Design review of the part built by this model. Coordinates are the model's own, in mm. A direction names the side the tool comes from. Give positions to 0.01 mm unless a question says otherwise; leave off trailing zeros. Write each loop counter-clockwise with the first axis right and the second up, starting at its lowest first coordinate (ties: lowest second). Pieces come first, ordered by that corner, then holes.
```python
from build123d import *

# Parameters (mm, degrees)
SKETCH1_W           = 1.5875
SKETCH1_H           = 40
SKETCH1_W_2         = 6.825
BOSS_EXTRUDE1_DEPTH = 1.5875
SKETCH1_3_W         = 1.5875
SKETCH1_3_H         = 40
BOSS_EXTRUDE2_DEPTH = 25
SKETCH2_W           = 10
SKETCH2_H           = 8
CUT_EXTRUDE1_DEPTH  = 11


with BuildPart() as part:
    # Sketch1 → Boss-Extrude1 (new body)
    with BuildSketch(Plane(origin=(0, 0, 0), x_dir=(1, 0, 0), z_dir=(0, 1, 0))):
        with Locations((-4.20625, 0)):
            Rectangle(SKETCH1_W, SKETCH1_H)
        Rectangle(SKETCH1_W_2, SKETCH1_H)
        with BuildLine():
            ThreePointArc((2.75, -10), (-1.944543648, -11.944543648), (0, -7.25))
            ThreePointArc((0, -7.25), (1.944543648, -8.055456352), (2.75, -10))
        make_face(mode=Mode.SUBTRACT)
        with BuildLine():
            ThreePointArc((2.75, 10), (1.944543648, 8.055456352), (0, 7.25))
            ThreePointArc((0, 7.25), (-1.944543648, 11.944543648), (2.75, 10))
        make_face(mode=Mode.SUBTRACT)
        with Locations((4.20625, 0)):
            Rectangle(SKETCH1_W, SKETCH1_H)
    extrude(amount=BOSS_EXTRUDE1_DEPTH)

    # Sketch1_3 → Boss-Extrude2 (add)
    with BuildSketch(Plane(origin=(0, 0, 0), x_dir=(1, 0, 0), z_dir=(0, 1, 0))):
        with Locations((-4.20625, 0)):
            Rectangle(SKETCH1_3_W, SKETCH1_3_H)
        with Locations((4.20625, 0)):
            Rectangle(SKETCH1_3_W, SKETCH1_3_H)
    extrude(amount=BOSS_EXTRUDE2_DEPTH)

    # Sketch2 → Cut-Extrude1 (cut, through all)
    with BuildSketch(Plane(origin=(5, 0, 0), x_dir=(0, 0, -1), z_dir=(1, 0, 0))):
        with Locations((-10, 5.5875)):
            Rectangle(SKETCH2_W, SKETCH2_H)
        with Locations((10, 5.5875)):
            Rectangle(SKETCH2_W, SKETCH2_H)
    extrude(amount=-CUT_EXTRUDE1_DEPTH, mode=Mode.SUBTRACT)


solid = part.part
```
(1) Consider section D-D, the plane x = -4. Give the boundary of the cut face in (y, z).
Resolved:
outline: (0, -20) - (25, -20) - (25, 20) - (0, 20) - close; hole (1.59, -15) - (9.59, -15) - (9.59, -5) - (1.59, -5) - close; hole (1.59, 5) - (9.59, 5) - (9.59, 15) - (1.59, 15) - close
(2) Consider section C-C, the plane z = 9.5. Give the boundary of the cut face in (x, y).
Resolved:
outline: (-5, 0) - (-2.7, 0) - (-2.7, 1.59) - (-5, 1.59) - close; (-5, 9.59) - (-3.41, 9.59) - (-3.41, 25) - (-5, 25) - close; (2.7, 0) - (5, 0) - (5, 1.59) - (2.7, 1.59) - close; (3.41, 9.59) - (5, 9.59) - (5, 25) - (3.41, 25) - close
(3) Consider section B-B, the plane y = 2.75. Give the boundary of the cut face in (x, z), then the cut area to 3 significant figures.
Resolved:
outline: (-5, -20) - (-3.41, -20) - (-3.41, -15) - (-5, -15) - close; (-5, -5) - (-3.41, -5) - (-3.41, 5) - (-5, 5) - close; (-5, 15) - (-3.41, 15) - (-3.41, 20) - (-5, 20) - close; (3.41, -20) - (5, -20) - (5, -15) - (3.41, -15) - close; (3.41, -5) - (5, -5) - (5, 5) - (3.41, 5) - close; (3.41, 15) - (5, 15) - (5, 20) - (3.41, 20) - close
area: 63.5 mm2
(4) Mouldability with a two-part tool opening along X and no side actions: class faces 1 (the face through (-4, 6, -5)), 2 (the face through (0, 1.588, 0)) as pulls with the +X half, pulls with the -X half, needs draft (parallel to the pull), parting line crosses it, or undercut.
Resolved:
face 1: needs draft
face 2: undercut
(5) To check wall thickness, follow L1, parallel to Z at x = 0, y = 0.6; L2, parallel to Z at x = 4.25, y = 8; L3, parallel to X at y = 21.75, z = 13. State the ranges of each line that lie inside material, in increasing order.
Resolved:
L1: z = -20 to -12.75, -7.25 to 7.25, 12.75 to 20
L2: z = -20 to -15, -5 to 5, 15 to 20
L3: x = -5 to -3.41, 3.41 to 5
(6) Tool access review of faces 3 (the face through (4, 11, -20)), 4 (the face through (-4, 6, 15)), 5 (the face through (-3.412, 16, 0)): name each direction out of +Z, -Z, +X, -X, +Y, -Y from which nothing blocks a thin tool from reaching the whole face with its end or side.
Resolved:
face 3: -Z, +X, -X, +Y, -Y
face 4: +X, -X
face 5: +Z, -Z, +Y
(7) Consider section A-A, the plane y = 15.5. Give the boundary of the cut face in (x, z), then the cut area to 3 significant figures.
Resolved:
outline: (-5, -20) - (-3.41, -20) - (-3.41, 20) - (-5, 20) - close; (3.41, -20) - (5, -20) - (5, 20) - (3.41, 20) - close
area: 127 mm2
